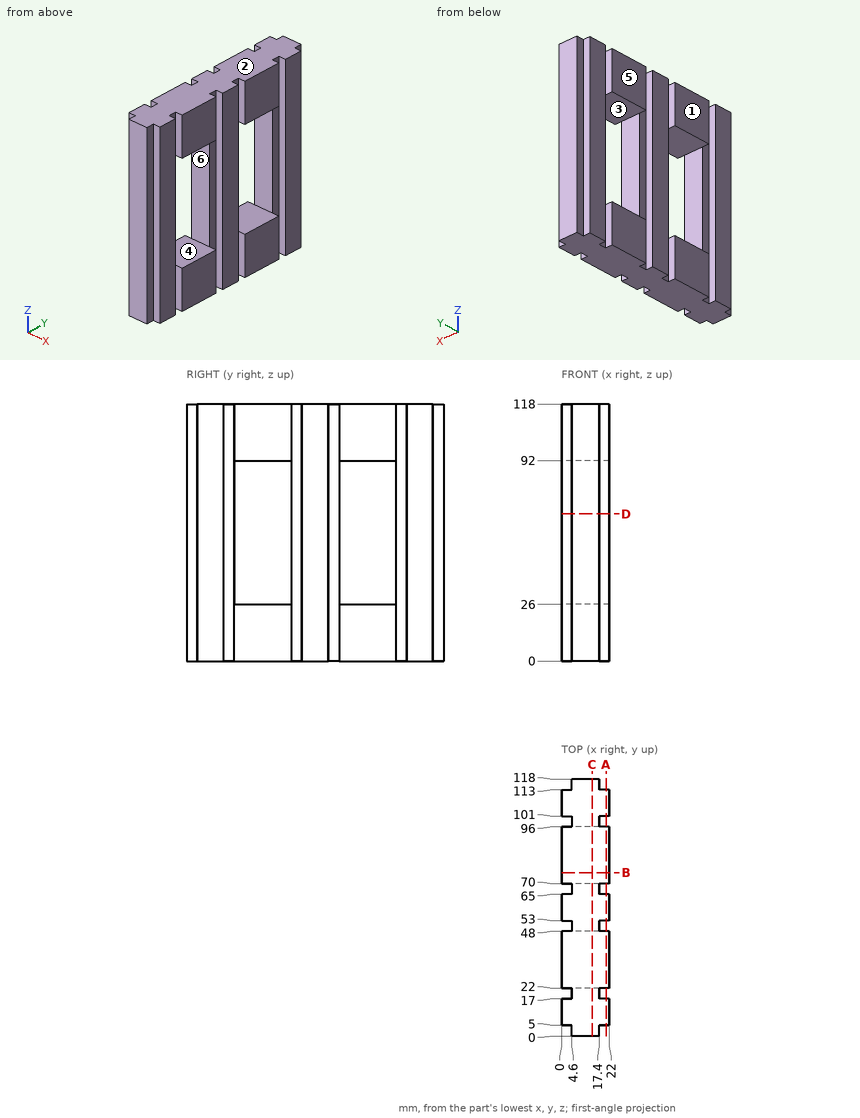
Input: dimensioned drawing with shaded views. Units: mm. Origin: part minimum x, y, z. A direction names the side the tool comes from. Give positions to 0.01 mm unless a question says otherwise; leave off trailing zeros. Loops run counter-clockwise (first coordinate to the right, second up) from the corner with the lowest first, then second, coordinate; pieces in that order, holes last. Notation, with made-up numbers: (-19, 8) -> (32, 8) arc R30 ccw to (32, 47) -> close; hole circle Ø10 at (-31, 78). An arc over 180 degrees is marked (long way). Use a Markdown table: item, result.
Q1. Section query B-B, the plane y = 75. Return the cut outline in (x, z), plus the area to 3 significant figures.
Entries:
| item | result |
|---|---|
| outline | (0, 0) -> (22, 0) -> (22, 26) -> (0, 26) -> close; (0, 92) -> (22, 92) -> (22, 118) -> (0, 118) -> close |
| area | 1,140 mm² |
Q2. Access query for the marked faces 5 and 6. Directions: +Z, -Z, +X, -X, +Y, -Y. A direction counts if a zero-diameter tool reaches every point of the face in a straight line with its end or side. Return the directions, or none.
Entries:
| item | result |
|---|---|
| face 5 | +Z, -Z, -X, +Y, -Y |
| face 6 | +X, -X |
Q3. Pull-direction query (Z, two-part tool) for the marked faces 1, 2, 3 and 4; classes: pulls with the +Z half, pulls with the -Z half, needs draft (parallel to the pull), parting line crosses it, or undercut.
Entries:
| item | result |
|---|---|
| face 1 | needs draft |
| face 2 | pulls with the +Z half |
| face 3 | undercut |
| face 4 | undercut |
Q4. Section query A-A, the plane x = 20.5. Return the cut outline in (y, z).
Entries:
| item | result |
|---|---|
| outline | (5, 0) -> (17, 0) -> (17, 118) -> (5, 118) -> close; (22, 0) -> (48, 0) -> (48, 26) -> (22, 26) -> close; (22, 92) -> (48, 92) -> (48, 118) -> (22, 118) -> close; (53, 0) -> (65, 0) -> (65, 118) -> (53, 118) -> close; (70, 0) -> (96, 0) -> (96, 26) -> (70, 26) -> close; (70, 92) -> (96, 92) -> (96, 118) -> (70, 118) -> close; (101, 0) -> (113, 0) -> (113, 118) -> (101, 118) -> close |
Q5. First-contact query: P1, Ø4, axis at y = 116.5, z = 60, coming from the +X side; P2, Ø1.4, axis at x = 1.5, z = 14, coming from the -Y side; P3, Ø3.5, axis at x = 19.5, z = 16, coming from the +Y side. Flat tips, straight axial feed; report the tip coordinate or a pass-through.
Entries:
| item | result |
|---|---|
| P1 | stops at x = 17.4 |
| P2 | stops at y = 5 |
| P3 | stops at y = 113 |
Q6. Ray query, probe 1 along Y at (x, z) = (15.75, 76.5); probe 2 along Y at (x, z) = (19.75, 111.5); probe 3 along Z at (x, y) = (13.25, 27.5). Return the intervals inside material, ascending. Write a range as from..to.
Entries:
| item | result |
|---|---|
| probe 1 | y = 0..22, 48..70, 96..118 |
| probe 2 | y = 5..17, 22..48, 53..65, 70..96, 101..113 |
| probe 3 | z = 0..26, 92..118 |
Q7. Section query C-C, the plane x = 14. Return the cut outline in (y, z).
Entries:
| item | result |
|---|---|
| outline | (0, 0) -> (118, 0) -> (118, 118) -> (0, 118) -> close; hole (22, 26) -> (48, 26) -> (48, 92) -> (22, 92) -> close; hole (70, 26) -> (96, 26) -> (96, 92) -> (70, 92) -> close |
Q8. Section query D-D, the plane z = 67.5. State how many separate pieces and enclosed holes the cut face has, plus the area to 3 significant figures.
Entries:
| item | result |
|---|---|
| separate pieces | 3 |
| enclosed holes | 0 |
| area | 1,180 mm² |
